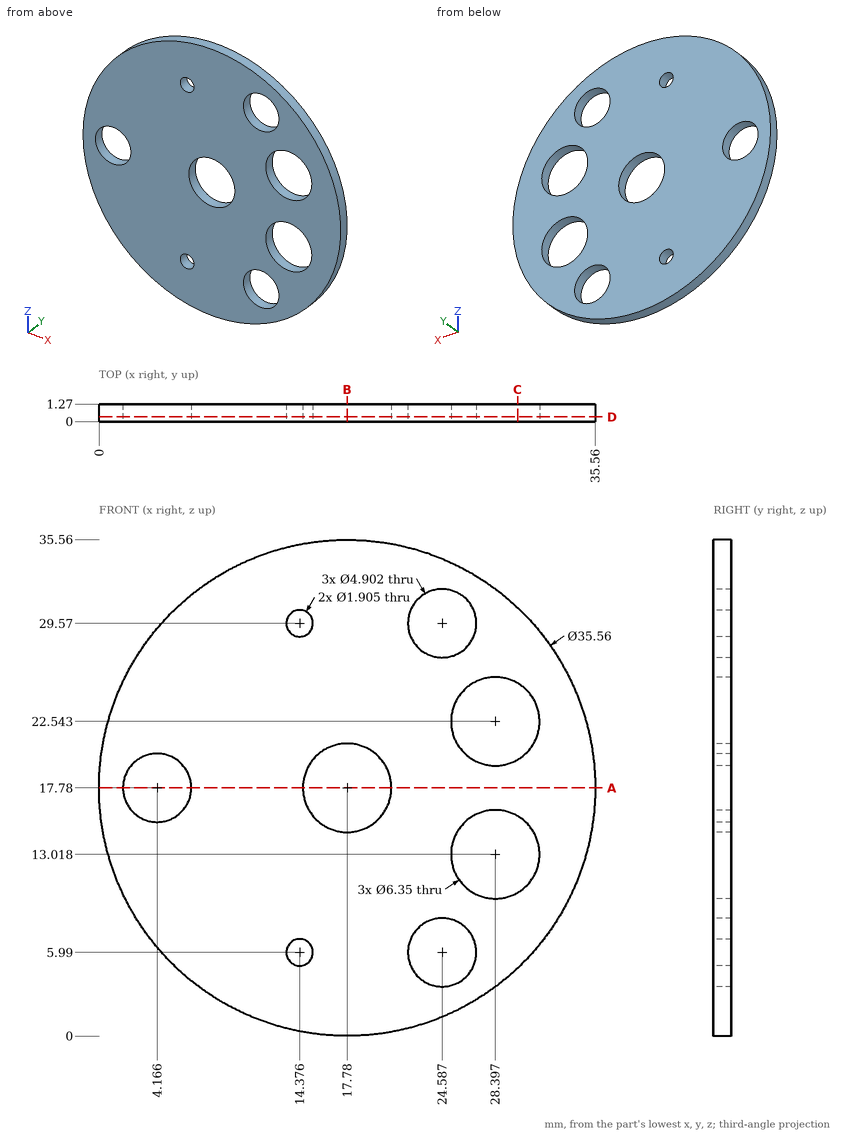
Source: three-view drawing plus pictorial views. Frame: mm from the lowest corner of the part. Coordinates: 2 decimals unless noted, no trailing zeros. Loops run counter-clockwise (first coordinate to the right, second up) from the corner with the lowest first, then second, coordinate; pieces in that order, holes last. Notation, with made-up numbers: (10, 79) -> (58, 79) arc R18 ccw to (58, 84) -> close; hole circle Ø1 at (38.25, 14.25). An arc over 180 degrees is marked (long way). One line per item, written item: value.
(1) Pin query (flat end, axial travel): pin 1 Ø2.5 at (x, z) = (14.38, 5.99) entering from -Y. Return the tip coordinate at first contact, or that it passes through.
Answer below:
pin 1: stops at y = 0
(2) Cut plane A-A (z = 17.78). Output: boundary loops of the cut face in (x, y) (1 decimal).
Answer below:
outline: (0, 0) -> (1.7, 0) -> (1.7, 1.3) -> (0, 1.3) -> close; (6.6, 0) -> (14.6, 0) -> (14.6, 1.3) -> (6.6, 1.3) -> close; (21, 0) -> (35.6, 0) -> (35.6, 1.3) -> (21, 1.3) -> close
(3) Cut plane D-D (y = 0.35). Give the number of separate pieces and of enclosed holes in the cut face, then the cut area to 3 significant figures.
Answer below:
separate pieces: 1
enclosed holes: 8
area: 836 mm2
(4) Cut plane C-C (x = 30). Output: boundary loops of the cut face in (y, z) (1 decimal).
Answer below:
outline: (0, 4.9) -> (1.3, 4.9) -> (1.3, 10.3) -> (0, 10.3) -> close; (0, 15.8) -> (1.3, 15.8) -> (1.3, 19.8) -> (0, 19.8) -> close; (0, 25.3) -> (1.3, 25.3) -> (1.3, 30.7) -> (0, 30.7) -> close
(5) Cut plane B-B (x = 17.78). Output: boundary loops of the cut face in (y, z) (1 decimal).
Answer below:
outline: (0, 0) -> (1.3, 0) -> (1.3, 14.6) -> (0, 14.6) -> close; (0, 21) -> (1.3, 21) -> (1.3, 35.6) -> (0, 35.6) -> close
(6) Ray query, line 1 along Z through (x, y) = (17.78, 1) (1 decimal); line 2 along Z through (x, y) = (28, 0.45); line 3 along X through (y, z) = (0.15, 4) (1 decimal). Return the intervals inside material, ascending.
Answer below:
line 1: z = 0 to 14.6, 21 to 35.6
line 2: z = 3.23 to 9.87, 16.17 to 19.39, 25.69 to 32.33
line 3: x = 6.5 to 23.2, 26 to 29
